```python
from build123d import *

# Parameters (mm, degrees)
SKETCH1_R                 = 25.4
BOSS_EXTRUDE1_DEPTH       = 6.35
SKETCH2_R                 = 9.525
BOSS_EXTRUDE2_DEPTH       = 6.35
SKETCH3_R                 = 4
CUT_EXTRUDE1_DEPTH        = 12.7
F_6_32_TAPPED_HOLE1_D     = 2.7051
F_6_32_TAPPED_HOLE1_DEPTH = 9.524
F_6_32_TAPPED_HOLE1_TIP   = 0.81269403


with BuildPart() as part:
    # Sketch1 → Boss-Extrude1 (new body)
    with BuildSketch(Plane.XY):
        Circle(SKETCH1_R)
    extrude(amount=BOSS_EXTRUDE1_DEPTH)

    # Sketch2 → Boss-Extrude2 (add)
    with BuildSketch(Plane.XY.offset(6.35)):
        Circle(SKETCH2_R)
    extrude(amount=BOSS_EXTRUDE2_DEPTH)

    # Sketch3 → Cut-Extrude1 (cut)
    with BuildSketch(Plane.XY.offset(12.7)):
        Circle(SKETCH3_R)
    extrude(amount=-CUT_EXTRUDE1_DEPTH, mode=Mode.SUBTRACT)

    # Sketch4 → Cut-Revolve1 (revolve, cut)
    with BuildSketch(Plane(origin=(0, 0, 0), x_dir=(1, 0, 0), z_dir=(0, 1, 0)), mode=Mode.PRIVATE) as cut_revolve1_sk:
        with BuildLine():
            Line((25.4, -6.35), (25.4, 0))
            ThreePointArc((25.4, 0), (22.225, -3.175), (25.4, -6.35))
        make_face()
    revolve(cut_revolve1_sk.sketch.rotate(Axis((0, 0, -6.424339231), (0, 0, 1)), 180), axis=Axis((0, 0, -6.424339231), (0, 0, 1)), mode=Mode.SUBTRACT)

    # #6-32 Tapped Hole1
    with Locations(Plane(origin=(0, 9.525, 9.525), x_dir=(1, 0, 0), z_dir=(0, 1, 0))):
        with Locations((0, 0)):
            Hole(F_6_32_TAPPED_HOLE1_D / 2, depth=F_6_32_TAPPED_HOLE1_DEPTH)
            with Locations((0, 0, -(F_6_32_TAPPED_HOLE1_DEPTH + F_6_32_TAPPED_HOLE1_TIP / 2))):  # 118° drill point
                Cone(0, F_6_32_TAPPED_HOLE1_D / 2, F_6_32_TAPPED_HOLE1_TIP, mode=Mode.SUBTRACT)


solid = part.part
```
Read the model definition and answer for the solid it produces. Units are mm, in the model's axes. A direction names the side the tool comes from. Round coordinates to 2 decimals unless told otherwise and drop trailing zeros. Write each loop counter-clockwise with the first axis right and the second up, starting at its lowest first coordinate (ties: lowest second). Pieces come first, ordered by that corner, then holes. Notation, with made-up numbers: (-27.75, -36) - (-20.75, -36) arc R20 cw to (-20.75, -2) - close; hole circle Ø11 at (-11, 9.25). An arc over 180 degrees is marked (long way). Use CSV: the item, a comma, the result in double quotes.
Q1. A tool of negligible diameter and unlimited length cuts with its end or side. For faces 1 (the flat face through (11, 0, 6.35)), 2 (the cylindrical face through (-0.867, -3.905, 6.439)), from which of +Z, -Z, +X, -X, +Y, -Y can it reach the whole face along a straight path? Write none if from no direction.
Values:
face 1,"+Z"
face 2,"+Z, -Z"
Q2. Each of these flat-tipped pins is pushed along its axis until it touches: pin 1 Ø1.5 at (x, y) = (5, -20) entering from +Z; pin 2 Ø4.5 at (x, z) = (0, 9.525) entering from -Y (3 decimals); pin 3 Ø6 at (x, y) = (10.5, -15.5) entering from -Z; pin 4 Ø1.5 at (x, z) = (-16.5, 3) entering from +Y. Where does it stop, or does it pass through?
Values:
pin 1,"stops at z = 6.35"
pin 2,"stops at y = -9.525"
pin 3,"stops at z = 0"
pin 4,"stops at y = 15.69"
Q3. Find section B-B, the plane y = 0. Write down the section's boundary in (x, z) (3 decimals).
Values:
outline,"(-25.4, 0) - (-4, 0) - (-4, 12.7) - (-9.525, 12.7) - (-9.525, 6.35) - (-25.4, 6.35) arc R3.175 cw to start; (4, 0) - (25.4, 0) arc R3.175 cw to (25.4, 6.35) - (9.525, 6.35) - (9.525, 12.7) - (4, 12.7) - close"
Q4. Find section D-D, the plane z = 4. Write down the section's boundary in (x, y), then the cut area to 3 significant figures.
Values:
outline,"circle Ø44.67 at (0, 0); hole circle Ø8 at (0, 0)"
area,"1,520 mm²"
Q5. Straight lines are drawn through the part: line 1 along Z through (x, y) = (0, 8); line 2 along Z through (x, y) = (18, -1.5); line 3 along Y through (x, z) = (0, 6). For each, find the intervals that lie inside material, in ascending order.
Values:
line 1,"z = 0 to 8.17, 10.88 to 12.7"
line 2,"z = 0 to 6.35"
line 3,"y = -23.95 to -4, 4 to 23.95"
Q6. Find section A-A, the plane x = 0. Write down the section's boundary in (y, z) (3 decimals), then the cut area to 3 significant figures.
Values:
outline,"(-25.4, 0) - (-4, 0) - (-4, 12.7) - (-9.525, 12.7) - (-9.525, 6.35) - (-25.4, 6.35) arc R3.175 cw to start; (4, 0) - (25.4, 0) arc R3.175 cw to (25.4, 6.35) - (9.525, 6.35) - (9.525, 8.172) - (4, 8.172) - close; (4, 10.878) - (9.525, 10.878) - (9.525, 12.7) - (4, 12.7) - close"
area,"295 mm²"
Q7. Find section C-C, the plane z = 12. Write down the section's boundary in (x, y) (3 decimals), then the cut area to 3 significant figures.
Values:
outline,"circle Ø19.05 at (0, 0); hole circle Ø8 at (0, 0)"
area,"235 mm²"
Q8. Determine the mould class of faces 3 (the flat face through (4, -2, 12.7)), 4 (the flat face through (5, 0, 0)), 5 (the cylindrical face through (0.176, 6.606, 8.184)) for opening direction Z: +Z half, -Z half, draft (parallel to the pull), parting line (faces both ways), or undercut.
Values:
face 3,"+Z half"
face 4,"-Z half"
face 5,"undercut"
